Geometry: final body of the model. Coordinates: model frame, mm. Face numbers are marked on the shaded views. Coordinates: 2 decimals unless noted, no trailing zeros. Order: outer loops, then holes, each group sorted by start corner. A loop starts at its lowest first (then second) coordinate and runs counter-clockwise, first axis right, second up. Notation, with made-up numbers: (27.5, 22.25) -> (39.5, 22.25) arc R17 ccw to (39.5, 35.25) -> close; hole circle Ø6 at (-7.5, -1). An arc over 180 degrees is marked (long way). Answer in a Markdown table with one row per item. Add a question column.
1) Pull-direction query (Y, two-part tool) for the marked faces 1, 2, 3 and 4; classes: +Y half, -Y half, draft (parallel to the pull), parting line (faces both ways), or undercut.
2) Section query A-A on y = -8.25. Return the cut outline in (x, z) (3 decimals), then the cut area to 3 significant figures.
3) Contact query for flat-ended pins moving along their axis: P1, Ø1.1, axis at x = 2.5, z = -20, coming from the -Y side; P2, Ø1, axis at x = 0.5, z = -25, coming from the -Y side; P3, Ø0.5, axis at x = -2.5, z = -17.5, coming from the -Y side. Output: stop coordinate, or through.
4) Section query D-D on z = -14. Return the cut outline in (x, y).
5) Ray query, line 1 (X direction, y = -2.75, z = -30); line 2 (Z direction, x = -0.4, y = -5.5); line 3 (Z direction, x = 0, y = -2.5). Return the intervals inside material, ascending. Write a range as from..to.
6) Section query B-B on z = -4. Return the cut outline in (x, y).
7) Section query C-C on z = -26. Return the cut outline in (x, y), then the cut area to 3 significant figures.
```python
from build123d import *

# Parameters (mm, degrees)
F1_DEPTH = 3
F3_D     = 3.3
F3_DEPTH = 10
F3_TIP   = 0.9914200214
F5_D     = 3.3
F5_DEPTH = 12
F5_TIP   = 0.9914200214
F7_DEPTH = 1


# Not quite as in the source:
# - a pattern or mirror of a feature is missing from the dataset's text; its kind, count and spacing are read off the source's solid
# - a feature names something its author has since deleted; it is built from what else it names


with BuildPart() as f1:
    # F0 (on Right) → F1 (new body, symmetric)
    with BuildSketch(Plane.YZ):
        Polygon((0, -55), (0, 0), (-30, 0), align=None)
    extrude(amount=F1_DEPTH, both=True)

    # F3
    with Locations(Plane(origin=(0, 0, 0), x_dir=(-1, 0, 0), z_dir=(0, 1, 0))):
        with Locations((0, -10), (0, -30)):
            Hole(F3_D / 2, depth=F3_DEPTH)
            with Locations((0, 0, -(F3_DEPTH + F3_TIP / 2))):  # 118° drill point
                Cone(0, F3_D / 2, F3_TIP, mode=Mode.SUBTRACT)

    # F5
    with Locations(Plane.XY):
        with Locations((0, -17)):
            Hole(F5_D / 2, depth=F5_DEPTH)
            with Locations((0, 0, -(F5_DEPTH + F5_TIP / 2))):  # 118° drill point
                Cone(0, F5_D / 2, F5_TIP, mode=Mode.SUBTRACT)

    # F6 (on face) → F7 (cut)
    with BuildSketch(Plane.YZ.offset(3)):
        with BuildLine():
            ThreePointArc((-2, -5), (-2.8786796564, -2.8786796564), (-5, -2))
            Line((-5, -2), (-21.5772890518, -2))
            ThreePointArc((-21.5772890518, -2), (-24.1569856595, -3.4686067089), (-24.2109757705, -6.436556392))
            Line((-24.2109757705, -6.436556392), (-7.6336867187, -36.8282529869))
            ThreePointArc((-7.6336867187, -36.8282529869), (-4.258737616, -38.2986761404), (-2, -35.3916965949))
            Line((-2, -35.3916965949), (-2, -5))
        make_face()
    f7 = extrude(amount=-F7_DEPTH, mode=Mode.SUBTRACT)

    # F7_copies: F7 across plane
    add(f7.mirror(Plane(origin=(0, 0, 0), x_dir=(0, 0, -1), z_dir=(-1, 0, 0))), mode=Mode.SUBTRACT)


solid = f1.part
```
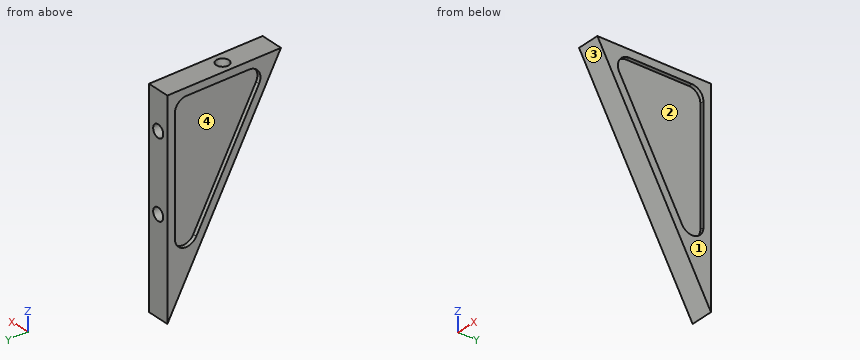
Result:
| question | item | result |
|---|---|---|
| 1 | face 1 | draft |
| 1 | face 2 | undercut |
| 1 | face 3 | -Y half |
| 1 | face 4 | undercut |
| 2 | outline | (-3, -39.875) -> (3, -39.875) -> (3, -35.698) -> (2, -35.698) -> (2, -2) -> (3, -2) -> (3, 0) -> (-3, 0) -> (-3, -2) -> (-2, -2) -> (-2, -35.698) -> (-3, -35.698) -> close; hole circle Ø3.3 at (0, -30); hole circle Ø3.3 at (0, -10) |
| 2 | area | 155 mm2 |
| 3 | P1 | y = -19.39 |
| 3 | P2 | y = -16.64 |
| 3 | P3 | y = -20.59 |
| 4 | outline | (-3, -22.36) -> (3, -22.36) -> (3, -20.09) -> (2, -20.09) -> (2, -2) -> (3, -2) -> (3, 0) -> (-3, 0) -> (-3, -2) -> (-2, -2) -> (-2, -20.09) -> (-3, -20.09) -> close |
| 5 | line 1 | -2..-1.65, 1.65..2 |
| 5 | line 2 | -44.92..-31.6, -28.4..-11.6, -8.4..0 |
| 5 | line 3 | -50.42..-31.65, -28.35..-11.65, -8.35..0 |
| 6 | outline | (-3, -27.82) -> (3, -27.82) -> (3, -24.41) -> (2, -24.41) -> (2, -2.17) -> (3, -2.17) -> (3, 0) -> (-3, 0) -> (-3, -2.17) -> (-2, -2.17) -> (-2, -24.41) -> (-3, -24.41) -> close; hole circle Ø3.3 at (0, -17) |
| 7 | outline | (-3, -15.82) -> (3, -15.82) -> (3, -13.54) -> (2, -13.54) -> (2, -2) -> (3, -2) -> (3, 0) -> (-3, 0) -> (-3, -2) -> (-2, -2) -> (-2, -13.54) -> (-3, -13.54) -> close |
| 7 | area | 71.8 mm2 |
